Geometry: see drawing. Coordinates: mm, zero at the bounding-box minimum. Round coordinates to 2 decimals unless told otherwise and drop trailing zeros. Order: outer loops, then holes, each group sorted by start corner. A loop starts at its lowest first (then second) coordinate and runs counter-clockwise, first axis right, second up. Notation, with made-up numbers: (-30, 40) -> (-3, 40) arc R23 ccw to (-3, 75) -> close; hole circle Ø10 at (81.5, 66). An arc over 180 degrees is marked (long way). Answer as CSV lines item,"result". Start each with the question number.
(1) Line query: line 1 along Y through (x, z) = (9.5, 36.5) (1 decimal); line 2 along Z through (x, y) = (33.5, 7.75) (1 decimal); line 3 along X through (y, z) = (1.5, 16) (1 decimal). Output: solid intervals per line, ascending. Write a range as from..to.
(2) Section query A-A (x = 20). Output: boundary loops of the cut face in (y, z) (1 decimal).
(3) Section query C-C (y = 1.5). Output: boundary loops of the cut face in (x, z), plus the area to 3 significant figures.
(4) Pull-direction query (Y, two-part tool) for the marked faces 1, 2 and 3; classes: +Y half, -Y half, draft (parallel to the pull), parting line (faces both ways), or undercut.
(5) Contact query for flat-ended pins moving along their axis: P1, Ø3, axis at x = 35, y = 2, coming from the -Z side (1 decimal); P2, Ø5, axis at y = 3.5, z = 23.5, coming from the +X side; P3, Ø3, axis at y = 4.5, z = 11, coming from the +X side (1 decimal). Output: stop coordinate, or through.
(6) Section query B-B (z = 20). Output: boundary loops of the cut face in (x, y) (1 decimal), plus the area to 3 significant figures.
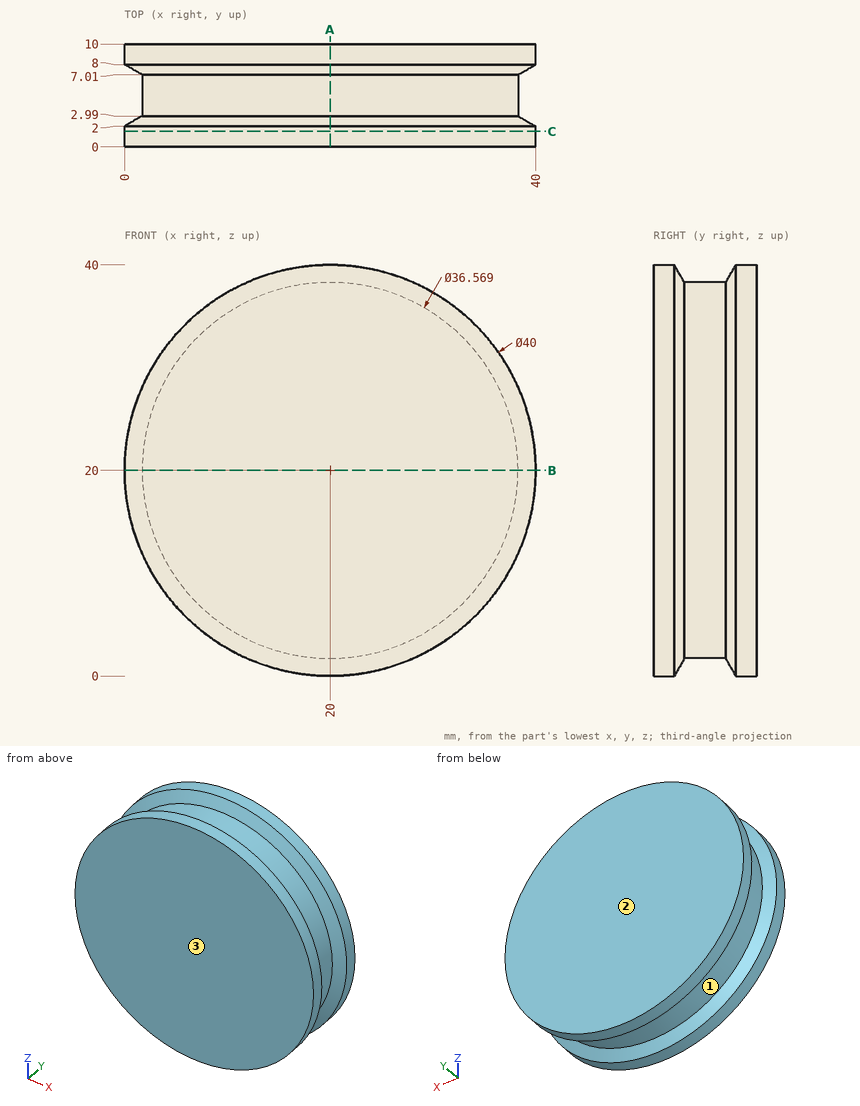
Answer block:
1,line 1,"0..2.3, 7.7..10"
1,line 2,"5.8..34.2"
1,line 3,"0.4..39.6"
2,outline,"(0, 0) -> (2, 0) -> (3, 1.7) -> (7, 1.7) -> (8, 0) -> (10, 0) -> (10, 40) -> (8, 40) -> (7, 38.3) -> (3, 38.3) -> (2, 40) -> (0, 40) -> close"
3,outline,"circle Ø40 at (20, 20)"
3,area,"1,260 mm2"
4,face 1,"undercut"
4,face 2,"+Y half"
4,face 3,"-Y half"
5,P1,"z = 5.2"
5,P2,"x = 39.94"
5,P3,"x = 36.7"
6,outline,"(0, 0) -> (40, 0) -> (40, 2) -> (38.3, 3) -> (38.3, 7) -> (40, 8) -> (40, 10) -> (0, 10) -> (0, 8) -> (1.7, 7) -> (1.7, 3) -> (0, 2) -> close"
6,area,"383 mm2"
